```python
from build123d import *

# Parameters (mm, degrees)
SKETCH_W        = 57.00014
SKETCH_H        = 57.00014
SKETCH_R        = 2.55
PAD_DEPTH       = 113.03
POCKET_DEPTH    = 107
SKETCH002_R     = 19.05
PAD001_DEPTH    = 1.6
SKETCH003_R     = 5
PAD002_DEPTH    = 24
FILLET_R        = 3.175
SKETCH004_W     = 30.604006
SKETCH004_H     = 8.312313
POCKET001_DEPTH = 20


with BuildPart() as part:
    # Sketch → Pad (new body)
    with BuildSketch(Plane.XY):
        Rectangle(SKETCH_W, SKETCH_H)
        with Locations((-23.5, 23.5)):
            Circle(SKETCH_R, mode=Mode.SUBTRACT)
        with Locations((23.5, 23.5)):
            Circle(SKETCH_R, mode=Mode.SUBTRACT)
        with Locations((-23.5, -23.5)):
            Circle(SKETCH_R, mode=Mode.SUBTRACT)
        with Locations((23.5, -23.5)):
            Circle(SKETCH_R, mode=Mode.SUBTRACT)
    extrude(amount=-PAD_DEPTH)

    # Sketch001 (on Face10 of Pad) → Pocket (cut)
    with BuildSketch(Plane(origin=(0, 0, -113.03), x_dir=(1, 0, 0), z_dir=(0, 0, -1))):
        with BuildLine():
            Line((-18.7375, 23.5), (-18.7375, 31.75))
            Line((-18.7375, 31.75), (-31.75, 31.75))
            Line((-31.75, 18.7375), (-31.75, 31.75))
            Line((-23.5, 18.7375), (-31.75, 18.7375))
            ThreePointArc((-23.5, 18.7375), (-20.190744, 20.190744), (-18.7375, 23.5))
        make_face()
        with BuildLine():
            Line((23.5, 18.7375), (31.75, 18.7375))
            Line((31.75, 18.7375), (31.75, 31.75))
            Line((18.7375, 31.75), (31.75, 31.75))
            Line((18.7375, 23.5), (18.7375, 31.75))
            ThreePointArc((18.7375, 23.5), (20.240641, 20.240641), (23.5, 18.7375))
        make_face()
        with BuildLine():
            Line((18.7375, -23.5), (18.7375, -31.75))
            Line((18.7375, -31.75), (31.75, -31.75))
            Line((31.75, -18.7375), (31.75, -31.75))
            Line((23.5, -18.7375), (31.75, -18.7375))
            ThreePointArc((23.5, -18.7375), (20.284094, -20.284094), (18.7375, -23.5))
        make_face()
        with BuildLine():
            Line((-23.5, -18.759919), (-31.75, -18.759919))
            Line((-31.75, -18.759919), (-31.75, -31.75))
            Line((-18.759919, -31.75), (-31.75, -31.75))
            Line((-18.759919, -23.5), (-18.759919, -31.75))
            ThreePointArc((-18.759919, -23.5), (-20.221862, -20.221862), (-23.5, -18.759919))
        make_face()
    extrude(amount=-POCKET_DEPTH, mode=Mode.SUBTRACT)

    # Sketch002 (on Face2 of Pocket) → Pad001 (join)
    with BuildSketch(Plane.XY):
        Circle(SKETCH002_R)
    extrude(amount=PAD001_DEPTH)

    # Sketch003 (on Face2 of Pad001) → Pad002 (join)
    with BuildSketch(Plane.XY):
        Circle(SKETCH003_R)
    extrude(amount=PAD002_DEPTH)

    # Fillet
    fillet_edges = [part.edges().sort_by_distance(p)[0] for p in [
        (28.50007, 28.50007, -3.015),
        (28.50007, -28.50007, -3.015),
        (-28.50007, 28.50007, -3.015),
        (-28.50007, -28.50007, -3.015),
    ]]
    fillet(fillet_edges, radius=FILLET_R)

    # Sketch004 (on Face34 of Fillet) → Pocket001 (cut)
    with BuildSketch(Plane.XY.offset(24)):
        with Locations((0, 8.728156)):
            Rectangle(SKETCH004_W, SKETCH004_H)
    extrude(amount=-POCKET001_DEPTH, mode=Mode.SUBTRACT)


solid = part.part
```
Input: part model. Units: mm. Frame: model coordinates. A direction names the side the tool comes from. Coordinates: 2 decimals unless noted, no trailing zeros. Loops run counter-clockwise (first coordinate to the right, second up) from the corner with the lowest first, then second, coordinate; pieces in that order, holes last.
Q1. Contact query for flat-ended pins moving along their axis: pin 1 (2.5 mm diameter, centred on x = -26.5, z = -78, fed in from +Y); pin 2 (5.5 mm diameter, centred on x = 27, z = -82.5, fed in from +Y); pin 3 (4 mm diameter, centred on y = -26.5, z = -64.5, fed in from -X). Output: stop coordinate, or through.
Results are:
pin 1: stops at y = 18.76
pin 2: stops at y = 18.74
pin 3: stops at x = -18.74
Q2. Section B-B, the plane z = -96. Return the cut outline in (x, y), and give its area (3 significant figures).
Results are:
outline: (-28.5, -18.74) - (-23.5, -18.74) arc R4.98 cw to (-18.74, -23.5) - (-18.74, -28.5) - (18.74, -28.5) - (18.74, -23.5) arc R5.19 cw to (23.5, -18.74) - (28.5, -18.74) - (28.5, 18.74) - (23.5, 18.74) arc R5.39 cw to (18.74, 23.5) - (18.74, 28.5) - (-18.76, 28.5) - (-18.76, 23.5) arc R5.02 cw to (-23.5, 18.76) - (-28.5, 18.76) - close
area: 2,890 mm2
Q3. Section A-A, the plane y = 0. Return the cut outline in (x, z), and give its area (3 significant figures).
Results are:
outline: (-28.5, -113.03) - (28.5, -113.03) - (28.5, 0) - (19.05, 0) - (19.05, 1.6) - (5, 1.6) - (5, 24) - (-5, 24) - (-5, 1.6) - (-19.05, 1.6) - (-19.05, 0) - (-28.5, 0) - close
area: 6,730 mm2
Q4. Line query: line 1 along Y through (x, z) = (23.5, -2.5); line 2 along X through (y, z) = (-23, -4); line 3 along Z through (x, y) = (-10, 5). Output: solid intervals per line, ascending.
Results are:
line 1: y = -28.5 to -26.05, -20.95 to 20.95, 26.05 to 28.5
line 2: x = -28.5 to -26, -21 to 21, 26 to 28.5
line 3: z = -113.03 to 1.6
Q5. Section C-C, the plane x = 15. Return the cut outline in (y, z).
Results are:
outline: (-28.5, -113.03) - (28.5, -113.03) - (28.5, 0) - (11.74, 0) - (11.74, 1.6) - (-11.74, 1.6) - (-11.74, 0) - (-28.5, 0) - close
Q6. Set-up query: faces 1 (the flat face through (18.738, 26, -60)), 2 (the flat face through (18.738, -26, -60)), 3 (the flat face through (4, -4, 1.6)). Return all of +Z, -Z, +X, -X, +Y, -Y with unobstructed straight access to the full face (end or side cutting, diameter ignored); none if empty.
Results are:
face 1: -Z, +X, +Y
face 2: -Z, +X, -Y
face 3: +Z
Q7. Section D-D, the plane y = -12. Return the cut outline in (x, z).
Results are:
outline: (-28.5, -113.03) - (28.5, -113.03) - (28.5, 0) - (14.8, 0) - (14.8, 1.6) - (-14.8, 1.6) - (-14.8, 0) - (-28.5, 0) - close
Q8. Mould query, pull axis X, two halves, no side actions, for faces 4 (the flat face through (-18.76, 26, -60)), 5 (the cylindrical face through (-25.4, 25.2, -3)), 6 (the flat face through (-26, 18.76, -60)), 7 (the cylindrical face through (27.55, -27.59, -3.06)). Classes: +X half, -X half, draft (parallel to the pull), parting line (faces both ways), or undercut.
Results are:
face 4: -X half
face 5: undercut
face 6: draft
face 7: +X half
